```python
from build123d import *

# Parameters (mm, degrees)
FILLET1_R = 5
FILLET2_R = 2
FILLET3_R = 5
FILLET4_R = 2


with BuildPart() as part:
    # Sketch2 → Revolve2 (revolve)
    with BuildSketch(Plane(origin=(0, 0, 0), x_dir=(0, 0, -1), z_dir=(1, 0, 0))):
        Polygon((-8, 2.5), (8, 2.5), (8, 7), (3, 7), (3, 32), (12.7, 32), (12.7, 36), (13, 36), (13, 50), (-13, 50), (-13, 36), (-12.7, 36), (-12.7, 32), (-3, 32), (-3, 7), (-8, 7), align=None)
    revolve(axis=Axis((0, 0, -5.520153215), (0, 0, 1)))

    # Fillet1
    fillet1_edges = [part.edges().sort_by_distance(p)[0] for p in [
        (0, -32, -3),
    ]]
    fillet(fillet1_edges, radius=FILLET1_R)

    # Fillet2
    fillet2_edges = [part.edges().sort_by_distance(p)[0] for p in [
        (0, -7, -3),
    ]]
    fillet(fillet2_edges, radius=FILLET2_R)

    # Fillet3
    fillet3_edges = [part.edges().sort_by_distance(p)[0] for p in [
        (0, -32, 3),
    ]]
    fillet(fillet3_edges, radius=FILLET3_R)

    # Fillet4
    fillet4_edges = [part.edges().sort_by_distance(p)[0] for p in [
        (0, -7, 3),
    ]]
    fillet(fillet4_edges, radius=FILLET4_R)


solid = part.part
```
Can you work these out from the model? Positions are in its coordinate system, mm. A direction names the side the tool comes from. Give positions to 0.01 mm unless a question says otherwise; leave off trailing zeros. Order: outer loops, then holes, each group sorted by start corner. A loop starts at its lowest first (then second) coordinate and runs counter-clockwise, first axis right, second up. Notation, with made-up numbers: M -14,-40 L 43,-40 A28 ccw 43,-19 Z; hole C 8,-34.5 d2. An arc over 180 degrees is marked long. Write item = value, one per line. Start each with the question number.
Q1. Will these pins go through, and if not, where does the flat tip stop? pin 1 Ø1.5 at (x, y) = (-23, 5) entering from +Z; pin 2 Ø5 at (y, z) = (3.5, -7.5) entering from +X; pin 3 Ø4 at (x, z) = (12, 9.5) entering from -Y; pin 4 Ø4 at (x, y) = (0, 0) entering from -Z.
Q2. I need wall thicknesses on probe 1 along Y at (x, z) = (0, -12.8); probe 2 along Y at (x, z) = (0, 9.45); probe 3 along X at (y, z) = (0, -2.25). Which ranges of each line are inside material? Lowest first, please. Write a range as [from, to].
Q3. Suppose I cut it at B-B (x = 44). Write out the boundary of the cut face in (y, z), plus the area to 3 significant figures.
Q4. Suppose I cut it at A-A (y = 40). Write out the boundary of the cut face in (x, z), plus the area to 3 significant figures.
Q5. We'd pull the mould along X, two halves only. Please class faces 4 (the flat face through (33, 22, 13)), 5 (the flat face through (0, 12, 3)), 6 (the cylindrical face through (-15.02, 47.69, 0.18)): pulls with the +X half, pulls with the -X half, needs draft (parallel to the pull), parting line crosses it, or undercut.
Q6. For faces 1 (the cylindrical face through (2.681, 6.466, -6.479)), 2 (the cylindrical face through (2.44, -0.54, -0.11)), 3 (the cylindrical face through (31.24, -6.94, 10.32)), which set-ups out of +Z, -Z, +X, -X, +Y, -Y let a thin tool reach every point of the face, with its end or its side?
Check result:
q1.pin_1 = 3
q1.pin_2 = 49.99
q1.pin_3 = -48.99
q1.pin_4 = through
q2.probe_1 = [-50, -36], [36, 50]
q2.probe_2 = [-50, -32], [32, 50]
q2.probe_3 = [-50, -2.5], [2.5, 50]
q3.outline = M -23.75,-13 L 23.75,-13 L 23.75,13 L -23.75,13 Z
q3.area = 1,230 mm2
q4.outline = M -30,-13 L 30,-13 L 30,13 L -30,13 Z
q4.area = 1,560 mm2
q5.face_4 = needs draft
q5.face_5 = undercut
q5.face_6 = parting line crosses it
q6.face_1 = -Z
q6.face_2 = +Z, -Z
q6.face_3 = +Z
